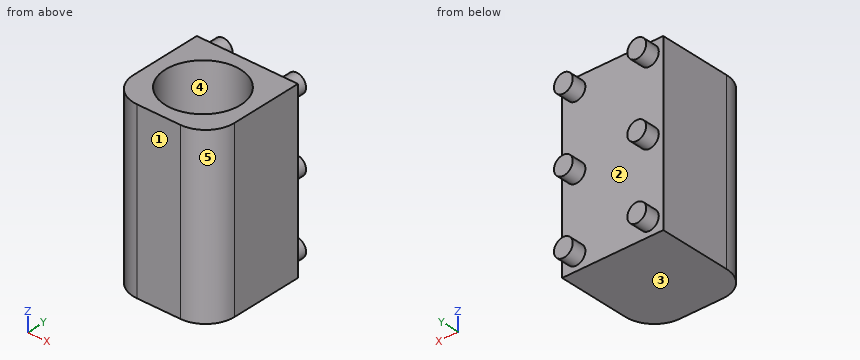
Autodesk Fusion 360 part; units mm, degrees
sketch "Sketch1" plane through (0, 0, 0) normal (0, 0, 1) x (1, 0, 0)
  line L0 (12.5427, 32.7282) -> (47.5427, 32.7282)
  line L1 (47.5427, 32.7282) -> (47.5427, 7.7282)
  line L2 (37.5427, -2.2718) -> (22.5427, -2.2718)
  line L3 (12.5427, 7.7282) -> (12.5427, 32.7282)
  line L4 (47.5427, 15.2282) -> (12.5427, 15.2282) construction
  line L5 (30.0427, 32.7282) -> (30.0427, 15.2282) construction
  circle A0 centre (30.0427, 15.2282) radius 13
  arc A1 (12.5427, 7.7282) -> (22.5427, -2.2718) centre (22.5427, 7.7282) ccw
  arc A2 (37.5427, -2.2718) -> (47.5427, 7.7282) centre (37.5427, 7.7282) ccw
  point P0 (12.5427, -2.2718)
  dimension "d1" = 35
  dimension "d2" = 35
  dimension "d4" = 26
  dimension "d21" = 10
extrude "Extrude2" add sketch "Sketch1" along normal blind 20 makes body 1
extrude "Extrude1" add sketch "Sketch1" along normal blind 2 separate body contours L0 L1 L2 L3 A1 A2 | A0 makes body 2
combine "Combine1" operation add target body 1 tool bodies 2
extrude "Extrude3" add 1 faces at (25.9943, 15.2712, 2) along direction (0, 0, 1) blind 3 on bodies 1 bodies 1
extrude "Extrude4" add 1 faces at (45.9943, 19.2074, 20) along direction (0, 0, 1) blind 40 on bodies 1 bodies 1
sketch "Sketch2" plane through (0, 32.7282, 0) normal (0, 1, 0) x (-1, 0, 0)
  line L0 (-12.5427, 0) -> (-12.5427, 60)
  line L1 (-12.5427, 60) -> (-47.5427, 60)
  line L2 (-47.5427, 60) -> (-47.5427, 0)
  line L3 (-47.5427, 0) -> (-12.5427, 0)
  line L4 (-47.5427, 60) -> (-12.5427, 60)
  line L5 (-12.5427, 60) -> (-12.5427, 0)
  line L6 (-12.5427, 0) -> (-47.5427, 0)
  line L7 (-47.5427, 0) -> (-47.5427, 60)
  circle A0 centre (-42.7427, 5) radius 3.25
  circle A1 centre (-17.3427, 5) radius 3.25
  circle A2 centre (-42.7427, 30.4) radius 3.25
  circle A3 centre (-17.3427, 30.4) radius 3.25
  circle A4 centre (-42.7427, 55.8) radius 3.25
  circle A5 centre (-17.3427, 55.8) radius 3.25
  dimension "d15" = 6.5
  dimension "d16" = 4.8
  dimension "d19" = 25.4
  dimension "d20" = 25.4
  dimension "d22" = 5
extrude "Extrude5" add sketch "Sketch2" along normal blind 5 contours A0 | A1 | A2 | A3 | A4 | A5 bodies 1
equation "PegWidth = 6.5 mm"
equation "HoleDistance = 25.4 mm"
equation "d15 = PegWidth"
equation "d16 = ( 35 mm - HoleDistance ) / 2"
equation "d20 = HoleDistance"
Part model, mm, in its own coordinate system. Face numbers are marked on the shaded views. A direction names the side the tool comes from. Round coordinates to 2 decimals unless told otherwise and drop trailing zeros. Loops run counter-clockwise (first coordinate to the right, second up) from the corner with the lowest first, then second, coordinate; pieces in that order, holes last.
1. Flat gauge pins, fed straight in: pin 1 (8 mm diameter, centred on x = 33.5, z = 46, fed in from +Y); pin 2 (2 mm diameter, centred on y = 5.5, z = 50.5, fed in from +X); pin 3 (1 mm diameter, centred on x = 33, y = 7, fed in from +Z). Where does each tip first touch, or does it go through?
Solutions:
pin 1: stops at y = 32.73
pin 2: stops at x = 47.47
pin 3: stops at z = 5
2. 3-axis set-ups, long thin cutter, end or side, ignore diameter. For the marked faces 1 and 2: which of +Z, -Z, +X, -X, +Y, -Y reach the whole face in a straight line?
Solutions:
face 1: +Z, -Z, +X, -X, -Y
face 2: +Y
3. Slice it at D-D (z = 6.5). Give the cut face in (x, y).
Solutions:
outline: (12.54, 7.73) arc R10 ccw to (22.54, -2.27) - (37.54, -2.27) arc R10 ccw to (47.54, 7.73) - (47.54, 32.73) - (45.63, 32.73) - (45.63, 37.73) - (39.86, 37.73) - (39.86, 32.73) - (20.23, 32.73) - (20.23, 37.73) - (14.46, 37.73) - (14.46, 32.73) - (12.54, 32.73) - close; hole circle Ø26 at (30.04, 15.23)
4. Slice it at A-A (y = 23). Give the cut face in (x, z).
Solutions:
outline: (12.54, 0) - (47.54, 0) - (47.54, 60) - (40.46, 60) - (40.46, 5) - (19.62, 5) - (19.62, 60) - (12.54, 60) - close
5. Slice it at C-C (z = 19.5). Give the cut face in (x, y), and give its area (3 significant figures).
Solutions:
outline: (12.54, 7.73) arc R10 ccw to (22.54, -2.27) - (37.54, -2.27) arc R10 ccw to (47.54, 7.73) - (47.54, 32.73) - (12.54, 32.73) - close; hole circle Ø26 at (30.04, 15.23)
area: 651 mm2
6. Slice it at B-B (x = 26). Give the cut face in (y, z).
Solutions:
outline: (-2.27, 0) - (32.73, 0) - (32.73, 60) - (27.58, 60) - (27.58, 5) - (2.87, 5) - (2.87, 60) - (-2.27, 60) - close
7. Drill centre lines: line 1 along Y through (x, z) = (30, 25.5); line 2 along Z through (x, y) = (17.5, 34); line 3 along Z through (x, y) = (41, 35.5). Where is each one in solid material? Low to high.
Solutions:
line 1: y = -2.27 to 2.23, 28.23 to 32.73
line 2: z = 1.75 to 8.25, 27.15 to 33.65, 52.55 to 59.05
line 3: z = 2.26 to 7.74, 27.66 to 33.14, 53.06 to 58.54
8. Two-plate mould, pull along Y, no slides. Class the marked faces 3, 4 and 5: pulls with the +Y half, pulls with the -Y half, needs draft (parallel to the pull), parting line crosses it, or undercut.
Solutions:
face 3: needs draft
face 4: undercut
face 5: pulls with the -Y half
